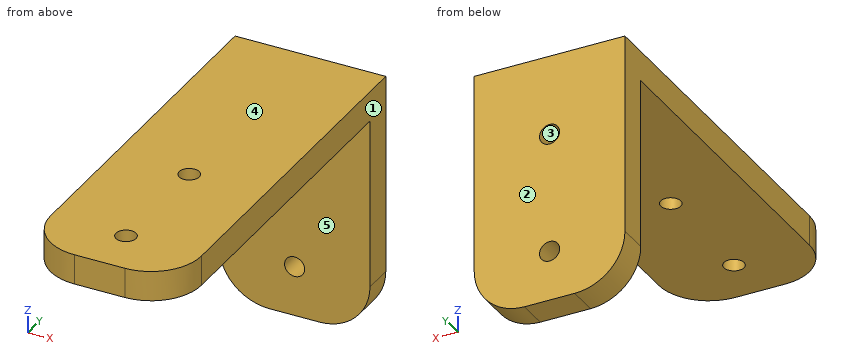
from build123d import *

# Parameters (mm, degrees)
SKETCH_1_R      = 1
EXTRUDE_1_DEPTH = 3
SKETCH_2_R      = 1
EXTRUDE_2_DEPTH = 3


with BuildPart() as part:
    # 草图1 → 凸台-拉伸1 (new body)
    with BuildSketch(Plane.XY):
        with BuildLine():
            Line((5, 0), (10, 0))
            ThreePointArc((10, 0), (13.535533906, 1.464466094), (15, 5))
            Line((15, 5), (15, 40))
            Line((15, 40), (0, 40))
            Line((0, 40), (0, 5))
            ThreePointArc((0, 5), (1.464466094, 1.464466094), (5, 0))
        make_face()
        with Locations((7.5, 5)):
            Circle(SKETCH_1_R, mode=Mode.SUBTRACT)
        with Locations((7.5, 17)):
            Circle(SKETCH_1_R, mode=Mode.SUBTRACT)
    extrude(amount=EXTRUDE_1_DEPTH)

    # 草图2 → 凸台-拉伸2 (add)
    with BuildSketch(Plane(origin=(0, 40, 0), x_dir=(-1, 0, 0), z_dir=(0, -1, 0))):
        with BuildLine():
            Line((-15, -3), (0, -3))
            Line((0, -3), (0, 17))
            ThreePointArc((0, 17), (-1.464466094, 20.535533906), (-5, 22))
            Line((-5, 22), (-10, 22))
            ThreePointArc((-10, 22), (-13.535533906, 20.535533906), (-15, 17))
            Line((-15, 17), (-15, -3))
        make_face()
        with Locations((-7.5, 17)):
            Circle(SKETCH_2_R, mode=Mode.SUBTRACT)
        with Locations((-7.5, 5)):
            Circle(SKETCH_2_R, mode=Mode.SUBTRACT)
    extrude(amount=EXTRUDE_2_DEPTH)


solid = part.part
The listing builds one solid part. Answer for the finished solid, in the listing's coordinates (mm). Face numbers are marked on the shaded views. A direction names the side the tool comes from. Give positions to 0.01 mm unless a question says otherwise; leave off trailing zeros. Write each loop counter-clockwise with the first axis right and the second up, starting at its lowest first coordinate (ties: lowest second). Pieces come first, ordered by that corner, then holes. Notation, with made-up numbers: (-27, -25.75) -> (21, -25.75) arc R13 cw to (21, -1.75) -> close; hole circle Ø4 at (26, 50.25). An arc over 180 degrees is marked (long way). One line per question, with ' | ' between items. Start each with the question number.
1. Section B-B (x = 7.5) is taken. Determine the outline of the cut face in (y, z).
2. Given pin 1 Ø6 at (x, y) = (13, 21) entering from -Z; pin 2 Ø1.8 at (x, y) = (7.5, 17) entering from -Z; pin 3 Ø2 at (x, z) = (6.5, -17) entering from -Y; pin 4 Ø6 at (x, z) = (2.5, -1.5) entering from -Y, each flat-ended and moving along its own axis, determine where each tip first touches the part or whether it passes through.
3. Section A-A (y = 17) is taken. Determine the outline of the cut face in (x, z), plus the area to 3 significant figures.
4. Section D-D (z = 0.5) is taken. Determine the outline of the cut face in (x, y).
5. For the marked faces 4 and 5, determine the directions among +Z, -Z, +X, -X, +Y, -Y from which every point of the face is accessible in a straight line to the end or side of a thin tool.
6. Section C-C (z = -5) is taken. Determine the outline of the cut face in (x, y), plus the area to 3 significant figures.
7. For a pull along X with two mould halves and no side action, classify the marked faces 1, 2 and 3 as pulls with the +X half, pulls with the -X half, needs draft (parallel to the pull), parting line crosses it, or undercut.
8. Find the intervals of material crossed by probe 1 along Z at (x, y) = (7.5, 39.4); probe 2 along Y at (x, z) = (7.5, 0.9); probe 3 along X at (y, z) = (38.75, -17), in increasing order.
Response values:
1) outline: (0, 0) -> (4, 0) -> (4, 3) -> (0, 3) -> close; (6, 0) -> (16, 0) -> (16, 3) -> (6, 3) -> close; (18, 0) -> (37, 0) -> (37, -4) -> (40, -4) -> (40, 3) -> (18, 3) -> close; (37, -22) -> (40, -22) -> (40, -18) -> (37, -18) -> close; (37, -16) -> (40, -16) -> (40, -6) -> (37, -6) -> close
2) pin 1: z = 0 | pin 2: through | pin 3: y = 37 | pin 4: y = 0
3) outline: (0, 0) -> (6.5, 0) -> (6.5, 3) -> (0, 3) -> close; (8.5, 0) -> (15, 0) -> (15, 3) -> (8.5, 3) -> close | area: 39.0 mm2
4) outline: (0, 5) arc R5 ccw to (5, 0) -> (10, 0) arc R5 ccw to (15, 5) -> (15, 40) -> (0, 40) -> close; hole circle Ø2 at (7.5, 5); hole circle Ø2 at (7.5, 17)
5) face 4: +Z, +X, -X, +Y, -Y | face 5: -Z, +X, -X, -Y
6) outline: (0, 37) -> (6.5, 37) -> (6.5, 40) -> (0, 40) -> close; (8.5, 37) -> (15, 37) -> (15, 40) -> (8.5, 40) -> close | area: 39.0 mm2
7) face 1: pulls with the +X half | face 2: needs draft | face 3: undercut
8) probe 1: -22 to -18, -16 to -6, -4 to 3 | probe 2: 0 to 4, 6 to 16, 18 to 40 | probe 3: 0 to 6.5, 8.5 to 15
